Check sheet for the modelled part. Datum: model origin and axes. Units: mm. A direction names the side the tool comes from. Round coordinates to 2 decimals unless told otherwise and drop trailing zeros. Write each loop counter-clockwise with the first axis right and the second up, starting at its lowest first coordinate (ties: lowest second). Pieces come first, ordered by that corner, then holes. Notation, with made-up numbers: (-11, 56.25) - (13, 56.25) arc R34 ccw to (13, 91.25) - close; hole circle Ø7 at (-31.75, 38). An arc over 180 degrees is marked (long way). Answer as a JSON object with one key per item and string values. Group by question number.
Item 1: Thickness scan on line 1 (X direction, y = 1.35, z = 5.5); line 2 (Z direction, x = 8.5, y = 1.3); line 3 (Z direction, x = -10, y = 1). Record the ranges inside material, lowest first.
Item 2: Sectioned sample at C-C on x = 15. Record the boundary of the cut face in (y, z), plus the area to 3 significant figures.
Item 3: Release check for a two-part mould opening along Z. For faces 3 (the flat face through (-3, 3, 3)), 4 (the cylindrical face through (-0.33, 1.48, -7.87)) record: pulls with the +Z half, pulls with the -Z half, needs draft (parallel to the pull), parting line crosses it, or undercut.
Item 4: Sectioned sample at B-B on y = 0.9. Count the separate pieces of the cut face and the enclosed holes in it, plus the area to 3 significant figures.
Item 5: Sectioned sample at A-A on z = 15. Record the boundary of the cut face in (x, y), plus the area to 3 significant figures.
Item 6: Gauge pin test, flat end, axial feed: P1, Ø1.6, axis at x = 15, z = 0, coming from the +Y side. Record the tip position at first contact, or that the pin passes through.
Item 7: Set-up check for faces 1 (the cylindrical face through (-1.5, 1.48, -0.07)), 2 (the cylindrical face through (0, 2, -14)): record each of +Z, -Z, +X, -X, +Y, -Y from which the full face is reachable in a straight line by a thin tool's end or side.
```python
from build123d import *

# Parameters (mm, degrees)
SKETCH_1_R               = 16.5
EXTRUDE_1_DEPTH          = 3
SKETCH_2_R               = 1
CUT_EXTRUDE_1_DEPTH      = 1.5
SKETCH_2_3_R             = 0.6
CUT_EXTRUDE_2_DEPTH      = 24.526580712
PATTERN_CIRCULAR_1_COUNT = 4
OTHER_1_OUTLINE_R        = 1.5
OTHER_1_DEPTH            = 3


# Read off the part's stored shape, not the designer's step: 填充阵列1
with BuildPart() as part:
    # 草图1 → 凸台-拉伸1 (new body)
    with BuildSketch(Plane(origin=(0, 0, 0), x_dir=(1, 0, 0), z_dir=(0, 1, 0))):
        with Locations(Location((0, 0, 0), (0, 0, 270))):
            Circle(SKETCH_1_R)
    extrude(amount=EXTRUDE_1_DEPTH)

    # 草图2 → 切除-拉伸1 (cut)
    with BuildSketch(Plane(origin=(0, 3, 0), x_dir=(1, 0, 0), z_dir=(0, 1, 0))):
        with Locations(Location((15, 0, 0), (0, 0, 270))):
            Circle(SKETCH_2_R)
    cut_extrude_1 = extrude(amount=-CUT_EXTRUDE_1_DEPTH, mode=Mode.SUBTRACT)

    # 草图2<3> → 切除-拉伸2 (cut, through all)
    with BuildSketch(Plane(origin=(0, 3, 0), x_dir=(1, 0, 0), z_dir=(0, 1, 0))):
        with Locations(Location((15, 0, 0), (0, 0, 270))):
            Circle(SKETCH_2_3_R)
    cut_extrude_2 = extrude(amount=-CUT_EXTRUDE_2_DEPTH, mode=Mode.SUBTRACT)

    # 阵列(圆周)1: 切除-拉伸1, 切除-拉伸2 ×4 about axis
    pattern_circular_1_axis = Axis((0, 0, 0), (0, 1, 0))
    add([cut_extrude_1.rotate(pattern_circular_1_axis, i * 360 / PATTERN_CIRCULAR_1_COUNT) for i in range(1, PATTERN_CIRCULAR_1_COUNT)], mode=Mode.SUBTRACT)
    add([cut_extrude_2.rotate(pattern_circular_1_axis, i * 360 / PATTERN_CIRCULAR_1_COUNT) for i in range(1, PATTERN_CIRCULAR_1_COUNT)], mode=Mode.SUBTRACT)

    # 填充阵列1 outline → 填充阵列1 (cut)
    with BuildSketch(Plane(origin=(0, 0, 0), x_dir=(1, 0, 0), z_dir=(0, 1, 0))):
        with Locations((0, 3.371e-06)):
            Circle(OTHER_1_OUTLINE_R)
        with Locations((-4.666904756, -9.333806141)):
            Circle(OTHER_1_OUTLINE_R)
        with Locations((0, -9.333806141)):
            Circle(OTHER_1_OUTLINE_R)
        with Locations((4.666904756, -9.333806141)):
            Circle(OTHER_1_OUTLINE_R)
        with Locations((9.333809512, -4.666901385)):
            Circle(OTHER_1_OUTLINE_R)
        with Locations((-9.333809512, 3.371e-06)):
            Circle(OTHER_1_OUTLINE_R)
        with Locations((0, 4.666908127)):
            Circle(OTHER_1_OUTLINE_R)
        with Locations((-9.333809512, 4.666908127)):
            Circle(OTHER_1_OUTLINE_R)
        with Locations((4.666904756, 4.666908127)):
            Circle(OTHER_1_OUTLINE_R)
        with Locations((-4.666904756, -4.666901385)):
            Circle(OTHER_1_OUTLINE_R)
        with Locations((-4.666904756, 3.371e-06)):
            Circle(OTHER_1_OUTLINE_R)
        with Locations((-9.333809512, -4.666901385)):
            Circle(OTHER_1_OUTLINE_R)
        with Locations((-4.666904756, 4.666908127)):
            Circle(OTHER_1_OUTLINE_R)
        with Locations((9.333809512, 3.371e-06)):
            Circle(OTHER_1_OUTLINE_R)
        with Locations((9.333809512, 4.666908127)):
            Circle(OTHER_1_OUTLINE_R)
        with Locations((4.666904756, 9.333812883)):
            Circle(OTHER_1_OUTLINE_R)
        with Locations((0, -4.666901385)):
            Circle(OTHER_1_OUTLINE_R)
        with Locations((4.666904756, 3.371e-06)):
            Circle(OTHER_1_OUTLINE_R)
        with Locations((-4.666904756, 9.333812883)):
            Circle(OTHER_1_OUTLINE_R)
        with Locations((4.666904756, -4.666901385)):
            Circle(OTHER_1_OUTLINE_R)
        with Locations((0, 9.333812883)):
            Circle(OTHER_1_OUTLINE_R)
    extrude(amount=OTHER_1_DEPTH, mode=Mode.SUBTRACT)


solid = part.part
```
Completed:
{
 "1": {"line 1": "-15.56 to -10.58, -8.09 to -5.91, -3.42 to -1.25, 1.25 to 3.42, 5.91 to 8.09, 10.58 to 15.56", "line 2": "-14.14 to -5.91, -3.42 to -1.25, 1.25 to 3.42, 5.91 to 14.14", "line 3": "-13.12 to -6.01, -3.32 to -1.34, 1.34 to 3.32, 6.01 to 13.12"},
 "2": {"outline": "(0, -6.87) - (3, -6.87) - (3, -1) - (1.5, -1) - (1.5, -0.6) - (0, -0.6) - close; (0, 0.6) - (1.5, 0.6) - (1.5, 1) - (3, 1) - (3, 6.87) - (0, 6.87) - close", "area": "36.4 mm²"},
 "3": {"face 3": "needs draft", "face 4": "undercut"},
 "4": {"separate pieces": "1", "enclosed holes": "25", "area": "702 mm²"},
 "5": {"outline": "(-6.87, 0) - (-0.6, 0) - (-0.6, 1.5) - (-1, 1.5) - (-1, 3) - (-6.87, 3) - close; (0.6, 0) - (6.87, 0) - (6.87, 3) - (1, 3) - (1, 1.5) - (0.6, 1.5) - close", "area": "36.4 mm²"},
 "6": {"P1": "y = 1.5"},
 "7": {"face 1": "+Y, -Y", "face 2": "+Y"}
}
